Work out the finished part from the listing and answer in its coordinate system (mm). A direction names the side the tool comes from. Give positions to 0.01 mm unless a question says otherwise; leave off trailing zeros. Write each loop counter-clockwise with the first axis right and the second up, starting at its lowest first coordinate (ties: lowest second). Pieces come first, ordered by that corner, then holes. Notation, with made-up numbers: (-20.75, 56) -> (-16.75, 56) arc R23 ccw to (-16.75, 94) -> close; hole circle Ø11 at (75, -34). An arc over 180 degrees is marked (long way). Use a Markdown table: item, result. Add a question column.
Q1. Section D-D, the plane x = 30 is taken. Give the vertices of the cut face in (y, z), plus the area to 3 significant figures.
Q2. Section B-B, the plane x = 1 is taken. Give the vertices of the cut face in (y, z) (3 decimals), plus the area to 3 significant figures.
Q3. Section A-A, the plane y = -1.5 is taken. Give the vertices of the cut face in (x, z).
Q4. Each of these flat-tipped pins is pushed along its axis until it touches: pin 1 Ø0.6 at (x, z) = (-28, 1) entering from -Y; pin 2 Ø1 at (y, z) = (29, 0.5) entering from +X; pin 3 Ø0.6 at (y, z) = (-35.5, 1) entering from -X. Where does it stop, or does it pass through?
Q5. For a pull along Y with two mould halves and no side action, classify faces 1 (the face through (-34, 5, 1)), 2 (the face through (5, -36, 1)), 3 (the face through (29, -35, 1)) as pulls with the +Y half, pulls with the -Y half, needs draft (parallel to the pull), parting line crosses it, or undercut.
Q6. Section C-C, the plane y = 27.5 is taken. Give the vertices of the cut face in (x, z).
Q7. Consider line 1 (Y direction, x = -1, z = 1.7) (3 decimals); line 2 (X direction, y = 5.5, z = 1.1); line 3 (X direction, y = 4, z = 1). Determine where each line is inside the solid, lowest interval first.
Q8. For faces 4 (the face through (33, -30, 1)), 5 (the face through (-33, -30, 1)), 6 (the face through (34, 25, 1)), 7 (the face through (-25, 36, 1)), 8 (the face through (0, -6.265, 1)), determine the directions among +Z, -Z, +X, -X, +Y, -Y from which every point of the face is accessible in a straight line to the end or side of a thin tool.
from build123d import *

# Parameters (mm, degrees)
SKETCH1_W           = 66
SKETCH1_H           = 70
BOSS_EXTRUDE1_DEPTH = 2
SKETCH2_W           = 2
SKETCH2_H           = 20
BOSS_EXTRUDE2_DEPTH = 2
SKETCH3_W           = 20
SKETCH3_H           = 2
BOSS_EXTRUDE3_DEPTH = 2
SKETCH4_W           = 7.1
SKETCH4_H           = 12.53
CUT_EXTRUDE1_DEPTH  = 10


with BuildPart() as part:
    # Sketch1 → Boss-Extrude1 (new body)
    with BuildSketch(Plane.XY):
        Rectangle(SKETCH1_W, SKETCH1_H)
    extrude(amount=BOSS_EXTRUDE1_DEPTH)

    # Sketch2 → Boss-Extrude2 (add)
    with BuildSketch(Plane(origin=(0, 0, 0), x_dir=(-1, 0, 0), z_dir=(0, 0, -1))):
        with Locations((34, -15)):
            Rectangle(SKETCH2_W, SKETCH2_H)
        with Locations((34, 15)):
            Rectangle(SKETCH2_W, SKETCH2_H)
        with Locations((-34, -15)):
            Rectangle(SKETCH2_W, SKETCH2_H)
        with Locations((-34, 15)):
            Rectangle(SKETCH2_W, SKETCH2_H)
    extrude(amount=-BOSS_EXTRUDE2_DEPTH)

    # Sketch3 → Boss-Extrude3 (add)
    with BuildSketch(Plane(origin=(0, 0, 0), x_dir=(-1, 0, 0), z_dir=(0, 0, -1))):
        with Locations((-15, 36)):
            Rectangle(SKETCH3_W, SKETCH3_H)
        with Locations((15, 36)):
            Rectangle(SKETCH3_W, SKETCH3_H)
        with Locations((-15, -36)):
            Rectangle(SKETCH3_W, SKETCH3_H)
        with Locations((15, -36)):
            Rectangle(SKETCH3_W, SKETCH3_H)
    extrude(amount=-BOSS_EXTRUDE3_DEPTH)

    # Sketch4 → Cut-Extrude1 (cut)
    with BuildSketch(Plane(origin=(0, 0, 0), x_dir=(-1, 0, 0), z_dir=(0, 0, -1))):
        Rectangle(SKETCH4_W, SKETCH4_H)
    extrude(amount=-CUT_EXTRUDE1_DEPTH, mode=Mode.SUBTRACT)


solid = part.part
Result set:
| question | item | result |
|---|---|---|
| 1 | outline | (-35, 0) -> (35, 0) -> (35, 2) -> (-35, 2) -> close |
| 1 | area | 140 mm2 |
| 2 | outline | (-35, 0) -> (-6.265, 0) -> (-6.265, 2) -> (-35, 2) -> close; (6.265, 0) -> (35, 0) -> (35, 2) -> (6.265, 2) -> close |
| 2 | area | 115 mm2 |
| 3 | outline | (-33, 0) -> (-3.55, 0) -> (-3.55, 2) -> (-33, 2) -> close; (3.55, 0) -> (33, 0) -> (33, 2) -> (3.55, 2) -> close |
| 4 | pin 1 | stops at y = -35 |
| 4 | pin 2 | stops at x = 33 |
| 4 | pin 3 | stops at x = -25 |
| 5 | face 1 | undercut |
| 5 | face 2 | needs draft |
| 5 | face 3 | pulls with the -Y half |
| 6 | outline | (-33, 0) -> (33, 0) -> (33, 2) -> (-33, 2) -> close |
| 7 | line 1 | y = -35 to -6.265, 6.265 to 35 |
| 7 | line 2 | x = -35 to -3.55, 3.55 to 35 |
| 7 | line 3 | x = -33 to -3.55, 3.55 to 33 |
| 8 | face 4 | +Z, -Z, +X, -Y |
| 8 | face 5 | +Z, -Z, -X, -Y |
| 8 | face 6 | +Z, -Z, +X, +Y |
| 8 | face 7 | +Z, -Z, -X, +Y |
| 8 | face 8 | +Z, -Z |
